```python
from build123d import *

# Parameters (mm, degrees)
F0_R     = 3.25
F1_DEPTH = 1.5


# Not quite as in the source:
# - ends of sketch curves that miss each other by under 0.0002 mm in the source are joined


with BuildPart() as f1:
    # F0 (on Top) → F1 (new body)
    with BuildSketch(Plane.XY):
        with BuildLine():
            ThreePointArc((11.5751507446, -4.5713014237), (14.9674174979, -3.4491015551), (18.5129609838, -3.00646439))
            ThreePointArc((18.5129609838, -3.00646439), (18.8578988072, -2.8554676082), (18.999681, -2.506641))
            Line((18.999681, -2.506641), (18.999681, -2.236416))
            ThreePointArc((18.999681, -2.236416), (19.1460678639, -1.882922365), (19.499512, -1.7364160286))
            Line((19.499512, -1.7364160286), (19.999851, -1.736246))
            ThreePointArc((19.999851, -1.736246), (20.3532944896, -1.5897392814), (20.499681, -1.236246))
            Line((20.499681, -1.236246), (20.499681, 0.013923))
            Line((20.499681, 0.013923), (20.499257, 1.263923))
            ThreePointArc((20.499257, 1.263923), (20.352690162, 1.6174265783), (19.999087, 1.7637529711))
            Line((19.999087, 1.7637529711), (19.499851, 1.763584))
            ThreePointArc((19.499851, 1.763584), (19.1461877186, 1.9099705104), (18.999681, 2.263584))
            Line((18.999681, 2.263584), (18.999681, 2.50664))
            ThreePointArc((18.999681, 2.50664), (18.8578988072, 2.8554666082), (18.5129609897, 3.0064636108))
            ThreePointArc((18.5129609897, 3.0064636108), (14.9674177085, 3.4491015077), (11.575151115, 4.5713012596))
            ThreePointArc((11.575151115, 4.5713012596), (9.5454328003, 4.9999983336), (7.5164170751, 4.5679878314))
            ThreePointArc((7.5164170751, 4.5679878314), (3.8419543275, 3.3757683124), (-0.000319, 2.9757689864))
            Line((-0.000319, 2.9757689864), (-18.499681, 2.999361))
            ThreePointArc((-18.499681, 2.999361), (-18.4999199994, 2.9993618408), (-18.5001589997, 2.9993619744))
            ThreePointArc((-18.5001589997, 2.9993619744), (-18.853403349, 2.8527463514), (-18.999681, 2.499362))
            Line((-18.999681, 2.499362), (-18.999681, 2.250339))
            ThreePointArc((-18.999681, 2.250339), (-19.1460675104, 1.8968457186), (-19.499511, 1.7503390289))
            Line((-19.499511, 1.7503390289), (-19.999851, 1.75017))
            ThreePointArc((-19.999851, 1.75017), (-20.3532944896, 1.6036632814), (-20.499681, 1.25017))
            Line((-20.499681, 1.25017), (-20.499681, 0))
            Line((-20.499681, 0), (-20.499256, -1.25))
            ThreePointArc((-20.499256, -1.25), (-20.3526895157, -1.6035032249), (-19.999087, -1.7498299714))
            Line((-19.999087, -1.7498299714), (-19.499851, -1.749661))
            ThreePointArc((-19.499851, -1.749661), (-19.1461877186, -1.8960475104), (-18.999681, -2.249661))
            Line((-18.999681, -2.249661), (-18.999681, -2.5))
            ThreePointArc((-18.999681, -2.5), (-18.8532343906, -2.8535533906), (-18.499681, -3))
            Line((-18.499681, -3), (-0.000319, -3))
            ThreePointArc((-0.000319, -3), (3.8532843758, -3.3991955476), (7.5432329323, -4.5798291546))
            ThreePointArc((7.5432329323, -4.5798291546), (9.5600895804, -4.9999888178), (11.5751507446, -4.5713014237))
        make_face()
        with Locations((9.549515, 0)):
            Circle(F0_R, mode=Mode.SUBTRACT)
    extrude(amount=F1_DEPTH)


solid = f1.part
```
Check sheet for the modelled part. Datum: model origin and axes. Units: mm. A direction names the side the tool comes from. Coordinates: 2 decimals unless noted, no trailing zeros. Loops run counter-clockwise (first coordinate to the right, second up) from the corner with the lowest first, then second, coordinate; pieces in that order, holes last.
1) Sectioned sample at C-C (x = 17). Record the boundary of the cut face in (y, z), and give its area (3 significant figures).
2) Gauge pin test, flat end, axial feed: pin 1 (0.6 mm diameter, centred on x = -19.5, z = 1, fed in from +Y). Record the tip position at first contact, or that the pin passes through.
3) Sectioned sample at D-D (x = -4). Record the boundary of the cut face in (y, z).
4) Sectioned sample at B-B (y = 0.5). Record the boundary of the cut face in (x, z).
5) Access from +Z, -Z, +X, -X, +Y, -Y to the whole of each face (thin tool, end or side, straight path). Record for faces 5 (the face through (9.6, 5, 0.7)), 6 (the face through (-9, -3, 1)).
6) Material ranges on probe 1 along X at (y, z) = (0.75, 1.05); probe 2 along X at (y, z) = (-2.5, 0.9); probe 3 along Y at (x, z) = (-11.5, 0.7), recorded low to high.
7) Release check for a two-part mould opening along X. For faces 1 (the face through (6.97, -1.98, 0.74)), 2 (the face through (0, 0, 0)), 3 (the face through (14.92, -3.46, 0.74)), 4 (the face through (3.8, -3.39, 0.74)) record: released by +X, released by -X, zero draft, split by the parting line, or undercut.
Check sheet entries:
1. outline: (-3.11, 0) - (3.11, 0) - (3.11, 1.5) - (-3.11, 1.5) - close
1. area: 9.33 mm2
2. pin 1: stops at y = 1.85
3. outline: (-3, 0) - (2.98, 0) - (2.98, 1.5) - (-3, 1.5) - close
4. outline: (-20.5, 0) - (6.34, 0) - (6.34, 1.5) - (-20.5, 1.5) - close; (12.76, 0) - (20.5, 0) - (20.5, 1.5) - (12.76, 1.5) - close
5. face 5: +Z, -Z, +Y
5. face 6: +Z, -Z, -X, -Y
6. probe 1: x = -20.5 to 6.39, 12.71 to 20.5
6. probe 2: x = -19 to 7.47, 11.63 to 19
6. probe 3: y = -3 to 2.99
7. face 1: undercut
7. face 2: zero draft
7. face 3: released by +X
7. face 4: released by -X
